Verification items for this drawing (mm, ordinates from the low corner). A direction names the side the tool comes from. Round coordinates to 2 decimals unless told otherwise and drop trailing zeros. Write each loop counter-clockwise with the first axis right and the second up, starting at its lowest first coordinate (ties: lowest second). Pieces come first, ordered by that corner, then holes.
Item 1: Scan lines: probe 1 along Y at (x, z) = (3.75, 4.5); probe 2 along Y at (x, z) = (1, 2); probe 3 along X at (y, z) = (4.25, 5.5) (3 decimals). Record each from-to range of solid material in increasing order.
Item 2: Cross-section at C-C (y = 2.5). Enter the section's corners in (x, z).
Item 3: Cross-section at D-D (x = 5.5). Enter the section's corners in (y, z), then the cut area to 4 significant figures.
Item 4: Depth check by flat-ended pin: P1, Ø3, axis at y = 3, z = 2.5, coming from the -X side; P2, Ø4, axis at x = 4, y = 1, coming from the -Z side; P3, Ø3, axis at x = 4.5, y = 4.5, coming from the +Z side. Enter the tip coordinate at first touch or a pass-through.
Item 5: Cross-section at B-B (z = 2.25). Enter the section's corners in (x, y).
Item 6: Cross-section at A-A (x = 2.5). Enter the section's corners in (y, z), then the cut area to 4 significant figures.
Item 7: Access from +Z, -Z, +X, -X, +Y, -Y to the whole of each face (thin tool, end or side, straight path). Record for the marked faces 1, 2, 3 and 4.
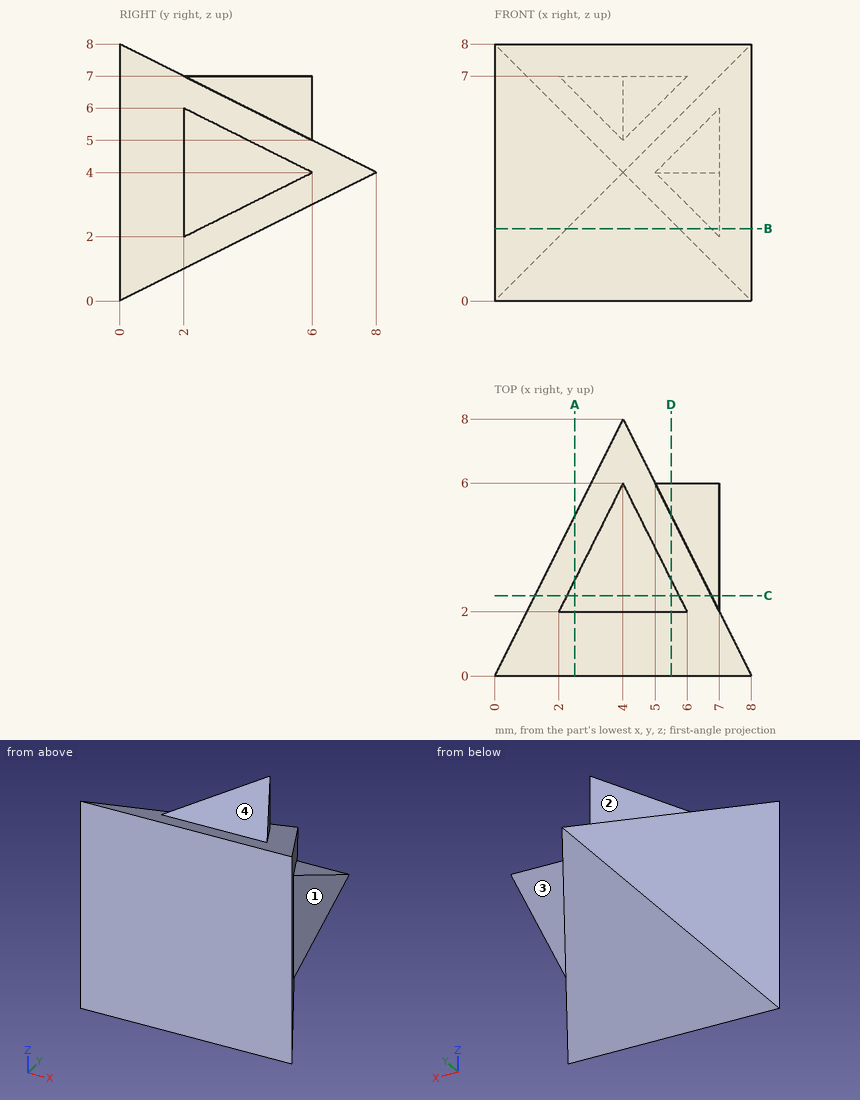
Resolved:
1. probe 1: y = 0 to 7
1. probe 2: y = 0 to 2
1. probe 3: x = 2.125 to 5.875
2. outline: (1.25, 1.25) - (6.75, 1.25) - (6.75, 2.25) - (7, 2.25) - (7, 5.75) - (6.75, 5.75) - (6.75, 6.75) - (5.75, 6.75) - (5.75, 7) - (2.25, 7) - (2.25, 6.75) - (1.25, 6.75) - close
3. outline: (0, 0) - (5, 2.5) - (5, 3.5) - (6, 4) - (5, 4.5) - (5, 5.5) - (3, 6.5) - (3, 7) - (2, 7) - (0, 8) - close
3. area: 28.25 mm2
4. P1: stops at x = 0.75
4. P2: stops at z = 0
4. P3: stops at z = 7
5. outline: (0, 0) - (8, 0) - (7, 2) - (7, 2.5) - (6.75, 2.5) - (5.75, 4.5) - (2.25, 4.5) - close
6. outline: (0, 0) - (5, 2.5) - (5, 5.5) - (3, 6.5) - (3, 7) - (2, 7) - (0, 8) - close
6. area: 27.75 mm2
7. face 1: +Z, -Z, +X, +Y
7. face 2: +Z, -X, +Y
7. face 3: -Z, +X, +Y
7. face 4: +Z, +X, -X, +Y
